Work out the finished part from the listing and answer in its coordinate system (mm). Give positions to 0.01 mm unless a question says otherwise; leave off trailing zeros. Order: outer loops, then holes, each group sorted by start corner. A loop starts at its lowest first (then second) coordinate and runs counter-clockwise, first axis right, second up.
```python
from build123d import *

# Parameters (mm, degrees)
F0_R     = 25.4
F0_R_2   = 15
F1_DEPTH = 6.35
F3_DEPTH = 12.701


with BuildPart() as f1:
    # F0 (on Top) → F1 (new body, symmetric)
    with BuildSketch(Plane.XY):
        Circle(F0_R)
        Circle(F0_R_2, mode=Mode.SUBTRACT)
    extrude(amount=F1_DEPTH, both=True)

    # F2 (on face) → F3 (cut, through all)
    with BuildSketch(Plane.XY.offset(6.35)):
        with BuildLine():
            ThreePointArc((0.254, -14.9978493125), (0, -15), (-0.254, -14.9978493125))
            Line((-0.254, -14.9978493125), (-0.254, -25.3987299682))
            ThreePointArc((-0.254, -25.3987299682), (0, -25.4), (0.254, -25.3987299682))
            Line((0.254, -25.3987299682), (0.254, -14.9978493125))
        make_face()
    extrude(amount=-F3_DEPTH, mode=Mode.SUBTRACT)


solid = f1.part
```
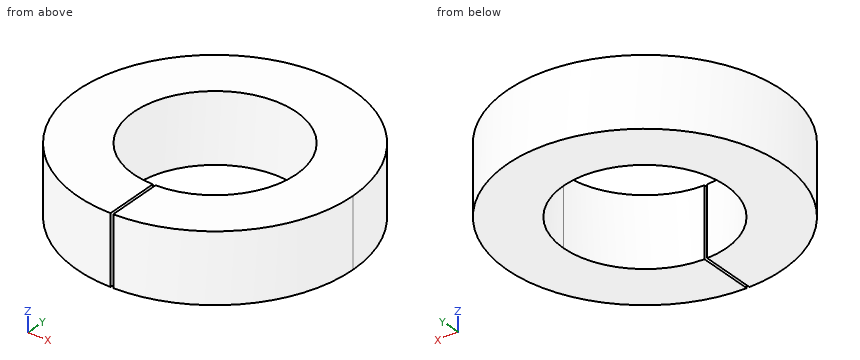
1. The part is cut by section C-C (z = 3.75). Write down the section's boundary in (x, y).
Findings below:
outline: (-0.25, -25.4) - (-0.25, -15) arc R15 cw (long way) to (0.25, -15) - (0.25, -25.4) arc R25.4 ccw (long way) to start
2. The part is cut by section D-D (x = -16.5). Write down the section's boundary in (y, z), then the cut area to 3 significant figures.
Findings below:
outline: (-19.31, -6.35) - (19.31, -6.35) - (19.31, 6.35) - (-19.31, 6.35) - close
area: 490 mm2
3. Given P1, Ø1.5, axis at y = -12.5, z = -1, coming from the -X side; P2, Ø3, axis at y = -18, z = 2.5, coming from the -X side; P3, Ø4, axis at y = -18, z = -1.5, coming from the +X side, each flat-ended and moving along its own axis, determine where each tip first touches the part or whether it passes through.
Findings below:
P1: stops at x = -22.52
P2: stops at x = -19.31
P3: stops at x = 19.73
4. The part is cut by section A-A (y = 3.5). Write down the section's boundary in (x, z), then the cut area to 3 significant figures.
Findings below:
outline: (-25.16, -6.35) - (-14.59, -6.35) - (-14.59, 6.35) - (-25.16, 6.35) - close; (14.59, -6.35) - (25.16, -6.35) - (25.16, 6.35) - (14.59, 6.35) - close
area: 269 mm2
5. Straight lines are drawn through the part: probe 1 along X at (y, z) = (0, -2); probe 2 along X at (y, z) = (-20.5, 3.25); probe 3 along Y at (x, z) = (0, 2.25). For each, find the intervals that lie inside material, in ascending order.
Findings below:
probe 1: x = -25.4 to -15, 15 to 25.4
probe 2: x = -15 to -0.25, 0.25 to 15
probe 3: y = 15 to 25.4
6. The part is cut by section B-B (x = -5). Write down the section's boundary in (y, z), then the cut area to 3 significant figures.
Findings below:
outline: (-24.9, -6.35) - (-14.14, -6.35) - (-14.14, 6.35) - (-24.9, 6.35) - close; (14.14, -6.35) - (24.9, -6.35) - (24.9, 6.35) - (14.14, 6.35) - close
area: 273 mm2
